from build123d import *

# Parameters (mm, degrees)
SKETCH2_W                = 28
SKETCH2_H                = 18
BOSS_EXTRUDE1_DEPTH      = 1.6
BOSS_EXTRUDE2_DEPTH      = 0.5
BOSS_EXTRUDE2_DEPTH_BACK = 9
SKETCH4_W                = 9.6
SKETCH4_H                = 11.5
SKETCH5_R                = 3.35
BOSS_EXTRUDE3_DEPTH      = 8
SKETCH6_W                = 4.7
SKETCH6_H                = 14.2
BOSS_EXTRUDE4_DEPTH      = 6
SKETCH7_R                = 1.9
CUT_EXTRUDE1_DEPTH       = 27.891262521
CHAMFER1_SIZE            = 2
SKETCH8_W                = 3.7
SKETCH8_H                = 13.2
CUT_EXTRUDE2_DEPTH       = 5


with BuildPart() as part:
    # Sketch2 → Boss-Extrude1 (new body)
    with BuildSketch(Plane(origin=(0, 0, 0), x_dir=(1, 0, 0), z_dir=(0, 1, 0))):
        Rectangle(SKETCH2_W, SKETCH2_H)
    extrude(amount=BOSS_EXTRUDE1_DEPTH)

    # Sketch4 → Boss-Extrude2 (add, two sides: drawn at the far end of the back side and taken through both)
    with BuildSketch(Plane(origin=(14, 0, 0), x_dir=(0, 0, -1), z_dir=(1, 0, 0)).offset(-BOSS_EXTRUDE2_DEPTH_BACK)):
        with Locations((0, 7.35)):
            Rectangle(SKETCH4_W, SKETCH4_H)
    extrude(amount=BOSS_EXTRUDE2_DEPTH + BOSS_EXTRUDE2_DEPTH_BACK)

    # Sketch5 → Boss-Extrude3 (add)
    with BuildSketch(Plane(origin=(14.5, 0, 0), x_dir=(0, 0, -1), z_dir=(1, 0, 0))):
        with Locations((0, 8)):
            Circle(SKETCH5_R)
    extrude(amount=BOSS_EXTRUDE3_DEPTH)

    # Sketch6 → Boss-Extrude4 (add)
    with BuildSketch(Plane(origin=(0, 1.6, 0), x_dir=(1, 0, 0), z_dir=(0, 1, 0))):
        with Locations((-3.55, -2.1)):
            Rectangle(SKETCH6_W, SKETCH6_H)
    extrude(amount=BOSS_EXTRUDE4_DEPTH)

    # Sketch7 → Cut-Extrude1 (cut, through all)
    with BuildSketch(Plane(origin=(0, 1.6, 0), x_dir=(1, 0, 0), z_dir=(0, 1, 0))):
        with Locations(Location((-10.1, 0, 0), (0, 0, 270))):
            Circle(SKETCH7_R)
    extrude(amount=-CUT_EXTRUDE1_DEPTH, mode=Mode.SUBTRACT)

    # Chamfer1
    chamfer1_edges = [part.edges().sort_by_distance(p)[0] for p in [
        (-14, 0.8, -9),
        (-14, 0.8, 9),
    ]]
    chamfer(chamfer1_edges, length=CHAMFER1_SIZE)

    # Sketch8 → Cut-Extrude2 (cut)
    with BuildSketch(Plane(origin=(0, 7.6, 0), x_dir=(1, 0, 0), z_dir=(0, 1, 0))):
        with Locations((-3.55, -2.1)):
            Rectangle(SKETCH8_W, SKETCH8_H)
    extrude(amount=-CUT_EXTRUDE2_DEPTH, mode=Mode.SUBTRACT)


solid = part.part
Geometry: final body of the model. Coordinates: model frame, mm. A direction names the side the tool comes from. Coordinates: 2 decimals unless noted, no trailing zeros. Loops run counter-clockwise (first coordinate to the right, second up) from the corner with the lowest first, then second, coordinate; pieces in that order, holes last. Notation, with made-up numbers: M 4,-7.75 L 57,-7.75 A16 ccw 57,10.25 Z; hole C 8,-17 d4. An arc over 180 degrees is marked long. One line per item, written item: value. Start each with the question number.
1) Pin query (flat end, axial travel): P1, Ø0.5, axis at y = 1, z = -2, coming from the +X side; P2, Ø1, axis at x = 5, y = 6, coming from the -Z side; P3, Ø5, axis at y = 6, z = 7.5, coming from the +X side. Return the tip coordinate at first contact, or that it passes through.
2) Reachability of faces 4 (the cylindrical face through (18.44, 4.73, 0.73)), 5 (the flat face through (-4, 5, 8.7)), 6 (the flat face through (10, 7, 4.8)) from +Z, -Z, +X, -X, +Y, -Y: full face, straight path, thin tool, end or side. Return the list, or none.
3) Cut plane A-A (x = -10.1). Return loops of the section in (y, z), then the cut area to 3 significant figures.
4) Cut plane B-B (y = 6.25). Return loops of the section in (x, z), then the cut area to 3 significant figures.
5) Cut plane D-D (x = 9). Return loops of the section in (y, z).
6) Material intervals for L1, parallel to X at y = 7, z = -1.75; L2, parallel to X at y = 0.5, z = 0; L3, parallel to X at y = 2.75, z = 3.25, sorted ascending. Write a range as from..to.
7) Cut plane C-C (z = 0). Return loops of the section in (x, y), then the cut area to 3 significant figures.
8) Draft query along X for faces 1 (the flat face through (-14, 1, 0)), 2 (the flat face through (-5.6, 7.6, 1.5)), 3 (the flat face through (-1.7, 5, 2)). Return one class per face: released by +X, released by -X, zero draft, split by the parting line, or undercut.
Evaluation:
1. P1: x = 14
1. P2: z = -4.8
1. P3: x = -1.2
2. face 4: +X
2. face 5: +Y
2. face 6: +Z, +X, +Y
3. outline: M 0,-9 L 1.6,-9 L 1.6,-1.9 L 0,-1.9 Z; M 0,1.9 L 1.6,1.9 L 1.6,9 L 0,9 Z
3. area: 22.7 mm^2
4. outline: M -5.9,-5 L -1.2,-5 L -1.2,9.2 L -5.9,9.2 Z; M 5,-4.8 L 14.5,-4.8 L 14.5,-2.86 L 22.5,-2.86 L 22.5,2.86 L 14.5,2.86 L 14.5,4.8 L 5,4.8 Z; hole M -5.4,-4.5 L -1.7,-4.5 L -1.7,8.7 L -5.4,8.7 Z
4. area: 155 mm^2
5. outline: M 0,-9 L 1.6,-9 L 1.6,-4.8 L 13.1,-4.8 L 13.1,4.8 L 1.6,4.8 L 1.6,9 L 0,9 Z
6. L1: -5.9..-5.4, -1.7..-1.2, 5..22.5
6. L2: -14..-12, -8.2..14
6. L3: -5.9..-5.4, -1.7..-1.2, 5..14.5
7. outline: M -14,0 L -12,0 L -12,1.6 L -14,1.6 Z; M -8.2,0 L 14,0 L 14,1.6 L 14.5,1.6 L 14.5,4.65 L 22.5,4.65 L 22.5,11.35 L 14.5,11.35 L 14.5,13.1 L 5,13.1 L 5,1.6 L -1.2,1.6 L -1.2,7.6 L -1.7,7.6 L -1.7,2.6 L -5.4,2.6 L -5.4,7.6 L -5.9,7.6 L -5.9,1.6 L -8.2,1.6 Z
7. area: 211 mm^2
8. face 1: released by -X
8. face 2: zero draft
8. face 3: undercut
